Part model, mm, in its own coordinate system. Coordinates: 2 decimals unless noted, no trailing zeros. Loops run counter-clockwise (first coordinate to the right, second up) from the corner with the lowest first, then second, coordinate; pieces in that order, holes last. Notation, with made-up numbers: M 18.5,12.5 L 51.5,12.5 A27 ccw 51.5,50.5 Z; hole C 53,-38 d1. An arc over 180 degrees is marked long. Use CSV: the item, a comma, the result in double quotes. Start each with the question number.
from build123d import *

# Parameters (mm, degrees)
F0_W     = 110
F0_H     = 20
F0_R     = 2.5
F0_R_2   = 0.5
F1_DEPTH = 20
F3_R     = 1.5
F4_DEPTH = 28.285271
F5_R     = 2.5
F5_R_2   = 0.5
F5_R_3   = 1.5
F6_DEPTH = 20.001


with BuildPart() as f1:
    # F0 (on Top) → F1 (new body)
    with BuildSketch(Plane.XY):
        Rectangle(F0_W, F0_H)
        with Locations((-50, 0)):
            Circle(F0_R, mode=Mode.SUBTRACT)
        with Locations((-44.9, 0)):
            Circle(F0_R_2, mode=Mode.SUBTRACT)
        with Locations((44.9, 0)):
            Circle(F0_R_2, mode=Mode.SUBTRACT)
        with Locations((50, 0)):
            Circle(F0_R, mode=Mode.SUBTRACT)
    extrude(amount=F1_DEPTH)

    # F3 (on face) → F4 (cut, through all)
    with BuildSketch(Plane(origin=(0, -15, 15), x_dir=(1, 0, 0), z_dir=(0, -0.707107, 0.707107))):
        with Locations((-34, 7.071068)):
            Circle(F3_R)
        with Locations((34, 7.071068)):
            Circle(F3_R)
    extrude(amount=-F4_DEPTH, mode=Mode.SUBTRACT)

    # F5 (on face) → F6 (cut, through all)
    with BuildSketch(Plane.XZ.offset(10)):
        with Locations((-44.9, 10)):
            Circle(F5_R)
        with Locations((44.9, 10)):
            Circle(F5_R)
        with Locations((-50, 10)):
            Circle(F5_R_2)
        with Locations((-29.933333, 10)):
            Circle(F5_R_3)
        with Locations((-14.966667, 10)):
            Circle(F5_R_3)
        with Locations((0, 10)):
            Circle(F5_R_3)
        with Locations((14.966667, 10)):
            Circle(F5_R_3)
        with Locations((29.933333, 10)):
            Circle(F5_R_3)
        with Locations((50, 10)):
            Circle(F5_R_2)
    extrude(amount=-F6_DEPTH, mode=Mode.SUBTRACT)


solid = f1.part
1. Pin check, flat tip, straight feed: pin 1 (3.5 mm diameter, centred on x = 14.97, z = 10, fed in from -Y). Stop position of the tip, or through.
2. Slice it at A-A, the plane x = 0. List the corners of the cut face in (y, z), and give its area (3 significant figures).
3. Wall check: probe 1 along X at (y, z) = (8.5, 1.75); probe 2 along X at (y, z) = (-8.5, 17.5); probe 3 along X at (y, z) = (3, 8). Give the ranges that are in metal, low to high.
4. Slice it at B-B, the plane y = -3.75. State how many separate pieces and enclosed holes the cut face has, and give its area (3 significant figures).
5. Two-plate mould, pull along X, no slides. Class faces 1 (the face through (-55, 0, 10)), 2 (the face through (-0.325, -0.14, 8.536)), 3 (the face through (-1, 0, 20)), 4 (the face through (-32.614, -0.546, 9.734)): pulls with the +X half, pulls with the -X half, needs draft (parallel to the pull), parting line crosses it, or undercut.
Found:
1,pin 1,"y = -10"
2,outline,"M -10,0 L 10,0 L 10,8.5 L -10,8.5 Z; M -10,11.5 L 10,11.5 L 10,20 L -10,20 Z"
2,area,"340 mm^2"
3,probe 1,"-55 to -35.49, -32.51 to 32.51, 35.49 to 55"
3,probe 2,"-55 to -35.32, -32.68 to 32.68, 35.32 to 55"
3,probe 3,"-55 to -46.4, -43.4 to -35.32, -32.68 to 32.68, 35.32 to 43.4, 46.4 to 55"
4,separate pieces,"1"
4,enclosed holes,"11"
4,area,"2,100 mm^2"
5,face 1,"pulls with the -X half"
5,face 2,"undercut"
5,face 3,"needs draft"
5,face 4,"undercut"
